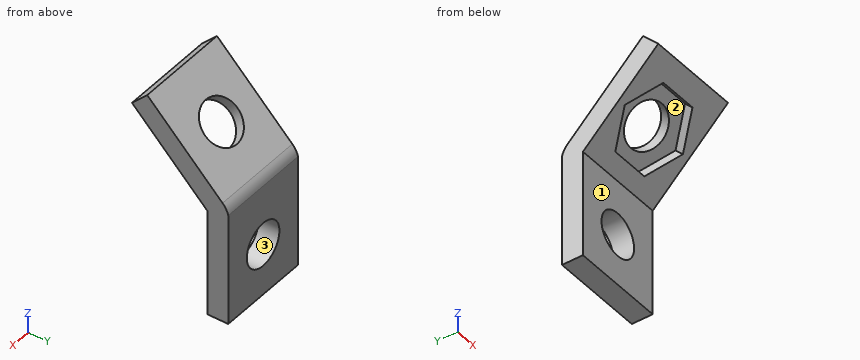
```python
from build123d import *

# Parameters (mm, degrees)
PAD014_DEPTH    = 9
SKETCH027_R     = 4.2
POCKET006_DEPTH = 5
SKETCH029_R     = 4.2
POCKET007_DEPTH = 5
POCKET008_DEPTH = 2


with BuildPart() as part:
    # Sketch026 → Pad014 (new body, symmetric)
    with BuildSketch(Plane.YZ):
        with BuildLine():
            Line((76.8243574995, 1.148527), (80.8243574995, 1.148527))
            Line((80.8243574995, 1.148527), (80.8243574995, 22.527915258))
            ThreePointArc((80.8243574995, 22.527915258), (80.4127450289, 23.566637908), (79.7371364968, 24.4565382849))
            Line((79.7371364968, 24.4565382849), (65.343272443, 38.8504023386))
            Line((65.343272443, 38.8504023386), (62.4304934457, 35.9376233413))
            Line((62.4304934457, 35.9376233413), (76.8243574995, 21.5437592876))
            Line((76.8243574995, 21.5437592876), (76.8243574995, 1.148527))
        make_face()
    extrude(amount=PAD014_DEPTH, both=True)

    # Sketch027 (on Face7 of Pad014) → Pocket006 (cut)
    with BuildSketch(Plane(origin=(0, 76.8243574995, 0), x_dir=(0, 0, -1), z_dir=(0, -1, 0))):
        with Locations((-11.01278, 0)):
            Circle(SKETCH027_R)
    extrude(amount=-POCKET006_DEPTH, mode=Mode.SUBTRACT)

    # Sketch029 (on Face6 of Pocket006) → Pocket007 (cut)
    with BuildSketch(Plane(origin=(0, 49.1840583935, 49.1840583935), x_dir=(0, 0.7071067812, -0.7071067812), z_dir=(0, -0.7071067812, -0.7071067812))):
        with Locations((29.346884, 0)):
            Circle(SKETCH029_R)
    extrude(amount=-POCKET007_DEPTH, mode=Mode.SUBTRACT)

    # Sketch030 (on Face6 of Pocket007) → Pocket008 (cut)
    with BuildSketch(Plane(origin=(0, 49.1840583935, 49.1840583935), x_dir=(0, 0.7071067812, -0.7071067812), z_dir=(0, -0.7071067812, -0.7071067812))):
        Polygon((22.846884, 3.7527767497), (22.846884, -3.7527767497), (29.346884, -7.5055534995), (35.846884, -3.7527767497), (35.846884, 3.7527767497), (29.346884, 7.5055534995), align=None)
    extrude(amount=-POCKET008_DEPTH, mode=Mode.SUBTRACT)


solid = part.part
```
CAD build for the part. Positions are in the model's coordinates, mm. Face numbers are marked on the shaded views. Coordinates: 2 decimals unless noted, no trailing zeros. Write each loop counter-clockwise with the first axis right and the second up, starting at its lowest first coordinate (ties: lowest second). Pieces come first, ordered by that corner, then holes. Notation, with made-up numbers: (-3, -30.5) -> (20, -30.5) arc R14 ccw to (20, -9.5) -> close; hole circle Ø2 at (59.5, 10.5). An arc over 180 degrees is marked (long way). Use CSV: the item, a comma, the result in double quotes. Start each with the question number.
Item 1: Wall check: probe 1 along Y at (x, z) = (-6, 15); probe 2 along X at (y, z) = (77, 9); probe 3 along Y at (x, z) = (2, 33.5). Give the ranges that are in metal, low to high.
Item 2: Band-saw the part on D-D, the plane z = 26. Write the cut outline in (x, y).
Item 3: Band-saw the part on B-B, the plane y = 79. Write the cut outline in (x, z).
Item 4: Band-saw the part on C-C, the plane x = 5.5. Write the cut outline in (y, z).
Item 5: Two-plate mould, pull along Y, no slides. Class the marked faces 1, 2 and 3: +Y half, -Y half, draft (parallel to the pull), parting line (faces both ways), or undercut.
Item 6: Band-saw the part on A-A, the plane x = -1.25. Write the cut outline in (y, z).
Item 7: Drop flat-ended pins along their axis: P1, Ø5, axis at x = 3.5, z = 31, coming from the +Y side; P2, Ø6, axis at y = 66.5, z = 31.5, coming from the +X side; P3, Ø9, axis at x = 0, z = 15, coming from the -Y side; P4, Ø3, axis at x = -6.5, y = 72, coming from the -Z side. Give the stop position or say it passes through.
Response values:
1,probe 1,"y = 76.82 to 80.82"
1,probe 2,"x = -9 to -3.69, 3.69 to 9"
1,probe 3,"y = 64.87 to 65.81, 67.7 to 69.78"
2,outline,"(-9, 72.37) -> (-5.52, 72.37) -> (-4.36, 75.2) -> (4.36, 75.2) -> (5.52, 72.37) -> (9, 72.37) -> (9, 78.19) -> (-9, 78.19) -> close"
3,outline,"(-9, 1.15) -> (9, 1.15) -> (9, 25.19) -> (-9, 25.19) -> close; hole circle Ø8.4 at (0, 11.01)"
4,outline,"(62.43, 35.94) -> (67.48, 30.89) -> (68.89, 32.3) -> (73.81, 27.39) -> (72.39, 25.98) -> (76.82, 21.54) -> (76.82, 1.15) -> (80.82, 1.15) -> (80.82, 22.53) arc R4.12 ccw to (79.74, 24.46) -> (65.34, 38.85) -> close"
5,face 1,"-Y half"
5,face 2,"undercut"
5,face 3,"draft"
6,outline,"(62.43, 35.94) -> (65.34, 33.03) -> (66.75, 34.44) -> (68.51, 32.68) -> (70.01, 34.18) -> (65.34, 38.85) -> close; (74.18, 27.01) -> (75.95, 25.25) -> (74.53, 23.84) -> (76.82, 21.54) -> (76.82, 15.02) -> (80.82, 15.02) -> (80.82, 22.53) arc R4.12 ccw to (79.74, 24.46) -> (75.68, 28.51) -> close; (76.82, 1.15) -> (80.82, 1.15) -> (80.82, 7) -> (76.82, 7) -> close"
7,P1,"stops at y = 75.69"
7,P2,"stops at x = 9"
7,P3,"stops at y = 76.82"
7,P4,"stops at z = 24.87"
